from build123d import *

# Parameters (mm, degrees)
F0_W     = 100
F0_H     = 100
F1_DEPTH = 6
F2_W     = 31.778058
F2_H     = 3.376421
F3_DEPTH = 3


with BuildPart() as f1:
    # F0 (on Top) → F1 (new body)
    with BuildSketch(Plane.XY):
        with Locations((1.715221, 12.071789)):
            Rectangle(F0_W, F0_H)
    extrude(amount=F1_DEPTH)

    # F2 (on face) → F3 (cut)
    with BuildSketch(Plane.XY.offset(6)):
        Polygon((12.313999, -35.849623), (12.313999, -37.928211), (17.676545, -37.928211), (17.676545, -19.563368), (23.833545, -19.563368), (23.833545, -35.849623), (27.706495, -35.849623), (49.851827, -35.849623), (49.851827, -32.274589), (49.851827, 58.491487), (48.064318, 58.491487), (24.429381, 58.491487), (24.429381, 55.909526), (24.429381, 26.912043), (26.812738, 26.912043), (46.078186, 26.912043), (46.078186, 29.494012), (46.078186, 53.724784), (43.496218, 53.724784), (29.196093, 53.724784), (29.196093, 51.540039), (29.196093, 31.480141), (31.182222, 31.480141), (41.311476, 31.480141), (41.311476, 34.062106), (41.311476, 49.156684), (39.523959, 49.156684), (32.969736, 49.156684), (32.969736, 46.773333), (32.969736, 35.65101), (34.558639, 35.65101), (37.736446, 35.65101), (37.736446, 37.239913), (34.558639, 37.239913), (34.558639, 46.773333), (39.523959, 46.773333), (39.523959, 34.062106), (31.182222, 34.062106), (31.182222, 51.540039), (43.496218, 51.540039), (43.496218, 29.494012), (26.812738, 29.494012), (26.812738, 55.909526), (48.064318, 55.909526), (48.064318, 25.323141), (-17.080707, 25.323141), (-19.464061, 25.323141), (-19.464061, -19.563368), (-19.464061, -21.549497), (-7.150063, -21.549497), (-4.17087, -21.549497), (-4.17087, 18.967528), (48.064318, 18.967528), (48.064318, -32.274589), (27.706495, -32.274589), (27.706495, -19.563368), (33.168349, -19.563368), (33.168349, -28.699558), (37.736446, -28.699558), (43.098994, -28.699558), (46.078186, -28.699558), (46.078186, 17.378626), (43.098994, 17.378626), (2.184742, 17.378626), (-2.383354, 17.378626), (-2.383354, -23.734238), (-21.847416, -23.734238), (-21.847416, 26.912043), (18.073771, 26.912043), (21.450188, 26.912043), (21.450188, 58.094267), (18.073771, 58.094267), (1.715221, 58.094267), (1.715221, 62.071789), (-2.780579, 62.071789), (-2.780579, 58.094267), (-2.780579, 54.717846), (18.073771, 54.717846), (18.073771, 30.487075), (-5.163935, 30.487075), (-5.163935, 41.212171), (1.787515, 41.212171), (1.787515, 35.253786), (4.766708, 35.253786), (15.690416, 35.253786), (15.690416, 38.232978), (15.690416, 52.135877), (12.115386, 52.135877), (12.115386, 38.232978), (4.766708, 38.232978), (4.766708, 41.212171), (4.766708, 44.787202), (-5.163935, 44.787202), (-8.34174, 44.787202), (-8.34174, 30.487075), (-16.683482, 30.487075), (-16.683482, 42.205233), (-20.0599, 42.205233), (-35.353091, 42.205233), (-35.353091, 38.431592), (-35.353091, -28.699558), (-32.373898, -28.699558), (-28.798867, -28.699558), (-28.798867, -25.323141), (-32.373898, -25.323141), (-32.373898, 33.267654), (-23.039093, 33.267654), (-23.039093, 35.849623), (-32.373898, 35.849623), (-32.373898, 38.431592), (-20.0599, 38.431592), (-20.0599, 30.487075), (-21.847416, 30.487075), (-26.415512, 30.487075), (-26.415512, -23.734238), (-26.415512, -27.309269), (-2.383354, -27.309269), (2.184742, -27.309269), (2.184742, 13.803595), (43.098994, 13.803595), (43.098994, -23.932852), (37.736446, -23.932852), (37.736446, -19.563368), (37.736446, -16.782787), (22.641867, -16.782787), (17.676545, -16.782787), (12.313999, -16.782787), (12.313999, -31.281527), (-39.126735, -31.281527), (-39.126735, 47.766395), (5.362547, 47.766395), (5.362547, 52.334495), (-10.725095, 52.334495), (-13.902901, 52.334495), (-39.126735, 52.334495), (-44.886511, 52.334495), (-44.886511, -31.281527), (-44.886511, -35.849623), align=None)
        Polygon((48.064318, 23.337012), (48.064318, 21.350883), (-4.17087, 21.350883), (-7.150063, 21.350883), (-7.150063, -19.563368), (-17.080707, -19.563368), (-17.080707, 23.337012), align=None, mode=Mode.SUBTRACT)
        Polygon((-13.902901, 56.902587), (-13.902901, 52.334495), (-10.725095, 52.334495), (-10.725095, 60.279008), (-13.902901, 60.279008), align=None)
        with Locations((-29.79193, 58.590797)):
            Rectangle(F2_W, F2_H)
        Polygon((17.676545, 0), (17.676545, -16.782787), (22.641867, -16.782787), (22.641867, 0), (25.32314, 0), (25.32314, -2.92954), (28.997479, -2.92954), (28.997479, 0), (32.969736, 0), (32.969736, 4.071564), (32.969736, 7.348676), (36.544766, 7.348676), (36.544766, -5.461854), (28.401639, -5.461854), (28.401639, -9.235498), (36.544766, -9.235498), (36.544766, -13.207756), (40.119801, -13.207756), (40.119801, 7.348676), (40.119801, 10.625788), (32.969736, 10.625788), (28.798867, 10.625788), (28.798867, 4.071564), (20.457124, 4.071564), (20.457124, 11.420241), (15.88903, 11.420241), (5.759772, 11.420241), (5.759772, 7.845208), (5.759772, 1.886822), (8.143128, 1.886822), (8.143128, 7.845208), (15.88903, 7.845208), (15.88903, 4.071564), (11.320934, 4.071564), (11.320934, 0), (4.965322, 0), (4.965322, -3.128153), (4.965322, -29.096784), (8.143129, -29.096784), (8.143129, -3.128153), (11.320934, -3.128153), (11.320934, -6.256306), (14.49874, -6.256306), (14.49874, 0), align=None)
    extrude(amount=-F3_DEPTH, mode=Mode.SUBTRACT)


solid = f1.part
Geometry check sheet. Reference: the model listing, model coordinates, mm. Give positions to 0.01 mm unless a question says otherwise; leave off trailing zeros.
1. Depth check by flat-ended pin: pin 1 (1.5 mm diameter, centred on x = 15.5, z = 4.5, fed in from -Y). Enter the tip coordinate at first touch or a pass-through.
Completed:
pin 1: stops at y = -16.78
2. Sectioned sample at A-A (z = 5). State how many separate pieces and enclosed holes the cut face has, then the cut area to 3 significant figures.
Completed:
separate pieces: 3
enclosed holes: 0
area: 5,250 mm2
3. Scan lines: line 1 (Y direction, x = -35.5, z = 5.4); line 2 (X direction, y = -31, z = 3.9); line 3 (Y direction, x = 21, z = 5.25). Record each from-to range of solid material in increasing order.
Completed:
line 1: y = -37.93 to -35.85, -31.28 to 47.77, 52.33 to 56.9, 60.28 to 62.07
line 2: x = -48.28 to -44.89, -39.13 to 12.31, 17.68 to 23.83, 27.71 to 48.06, 49.85 to 51.72
line 3: y = -37.93 to -19.56, 4.07 to 13.8, 17.38 to 18.97, 21.35 to 23.34, 25.32 to 26.91, 58.09 to 62.07
4. Draft check along Y on faces 1 (the face through (23.834, -28, 5)), 2 (the face through (37, 55.91, 5)), 3 (the face through (1, -37.928, 3)). Enter one of: pulls with the +Y half, pulls with the -Y half, needs draft (parallel to the pull), parting line crosses it, or undercut.
Completed:
face 1: undercut
face 2: undercut
face 3: pulls with the -Y half
